Build history of the part. All positions in model axes, mm. Round coordinates to 2 decimals unless told otherwise and drop trailing zeros. Loops run counter-clockwise (first coordinate to the right, second up) from the corner with the lowest first, then second, coordinate; pieces in that order, holes last.
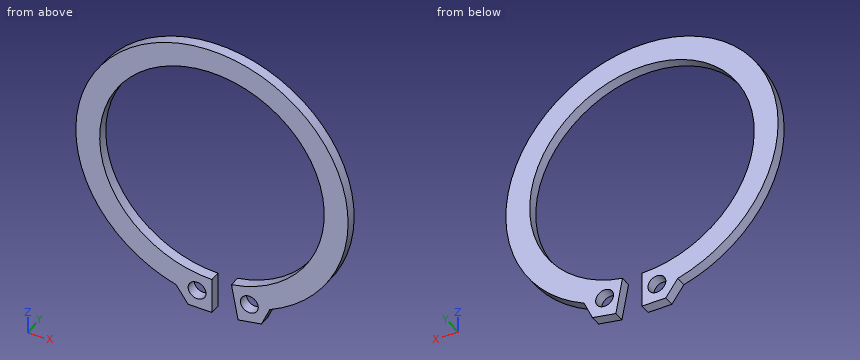
from build123d import *

# Parameters (mm, degrees)
BOSS_EXTRUDE1_DEPTH = 0.889
SKETCH4_R           = 0.75
CUT_EXTRUDE2_DEPTH  = 0.889


with BuildPart() as part:
    # Sketch1 → Boss-Extrude1 (new body)
    with BuildSketch(Plane(origin=(0, 0, 0), x_dir=(1, 0, 0), z_dir=(0, 1, 0))):
        with BuildLine():
            Line((0, 12.414484685), (-2, 12.414484685))
            Line((-2, 12.414484685), (-3, 11.013194842))
            ThreePointArc((-3, 11.013194842), (-0.984968358, -11.371908281), (4.848914718, 10.333367635))
            Line((4.848914718, 10.333367635), (4.155731478, 11.908137913))
            Line((4.155731478, 11.908137913), (2.189008602, 12.271457509))
            Line((2.189008602, 12.271457509), (1.634808109, 9.271457509))
            ThreePointArc((1.634808109, 9.271457509), (-0.820526405, -9.378659729), (0, 9.414484685))
            Line((0, 9.414484685), (0, 12.414484685))
        make_face()
    extrude(amount=BOSS_EXTRUDE1_DEPTH)

    # Sketch4 → Cut-Extrude2 (cut)
    with BuildSketch(Plane(origin=(0, 0.889, 0), x_dir=(1, 0, 0), z_dir=(0, 1, 0))):
        with Locations(Location((-1.25, 10.872808275, 0), (0, 0, 270))):
            Circle(SKETCH4_R)
        with Locations(Location((3.134471061, 10.508444008, 0), (0, 0, 270))):
            Circle(SKETCH4_R)
    extrude(amount=-CUT_EXTRUDE2_DEPTH, mode=Mode.SUBTRACT)


solid = part.part
(1) Slice it at B-B on x = -8. List the corners of the cut face in (y, z).
Responses:
outline: (0, -8.14) - (0.89, -8.14) - (0.89, -4.96) - (0, -4.96) - close; (0, 4.96) - (0.89, 4.96) - (0.89, 8.14) - (0, 8.14) - close
(2) Slice it at A-A on z = 0. List the corners of the cut face in (x, y), plus the area to 3 significant figures.
Responses:
outline: (-11.41, 0) - (-9.41, 0) - (-9.41, 0.89) - (-11.41, 0.89) - close; (9.41, 0) - (11.41, 0) - (11.41, 0.89) - (9.41, 0.89) - close
area: 3.56 mm2
(3) Slice it at C-C on x = -1.25. List the corners of the cut face in (y, z), plus the area to 3 significant figures.
Responses:
outline: (0, -12.41) - (0.89, -12.41) - (0.89, -11.62) - (0, -11.62) - close; (0, -10.12) - (0.89, -10.12) - (0.89, -9.33) - (0, -9.33) - close; (0, 9.33) - (0.89, 9.33) - (0.89, 11.35) - (0, 11.35) - close
area: 3.20 mm2
(4) Slice it at D-D on y = 0.2. List the corners of the cut face in (x, z).
Responses:
outline: (-3, -11.01) - (-2, -12.41) - (0, -12.41) - (0, -9.41) arc R9.41 cw (long way) to (1.63, -9.27) - (2.19, -12.27) - (4.16, -11.91) - (4.85, -10.33) arc R11.41 ccw (long way) to start; hole circle Ø1.5 at (-1.25, -10.87); hole circle Ø1.5 at (3.13, -10.51)
(5) Probe line 1 (Z direction, x = -1, y = 0.7); line 2 (X direction, y = 0.55, z = -10.5); line 3 (X direction, y = 0.35, z = 7.25). List the from-to ranges inside material, lowest first.
Responses:
line 1: z = -12.41 to -11.58, -10.17 to -9.36, 9.36 to 11.37
line 2: x = -4.48 to -1.9, -0.6 to 0, 1.86 to 2.38, 3.88 to 4.78
line 3: x = -8.82 to -6.01, 6.01 to 8.82
